The model under review builds one solid part; all positions refer to its coordinate system, in mm. Round coordinates to 2 decimals unless told otherwise and drop trailing zeros. Loops run counter-clockwise (first coordinate to the right, second up) from the corner with the lowest first, then second, coordinate; pieces in that order, holes last. Notation, with made-up numbers: M 47,-33 L 65,-33 A17 ccw 65,0 Z; hole C 18.25,48 d9. An arc over 180 degrees is marked long. Return JSON: item names as keys, results as strings. Group by question number.
Q1. To check wall thickness, follow line 1 along Y through (x, z) = (0, 7.5); line 2 along X through (y, z) = (3.5, 22.5); line 3 along X through (y, z) = (-24, 10.5). State the ranges of each line that lie inside material, in increasing order.
Q2. Consider section D-D (z = 8). State the section outline as (x, y) points.
Q3. Clearance check with flat-ended pins moving along their axes: pin 1 Ø6 at (y, z) = (-13, 22) entering from +X; pin 2 Ø4 at (x, y) = (10.5, 21) entering from -Z; pin 3 Ø5 at (x, y) = (0, 0) entering from -Z; pin 4 Ø1.5 at (y, z) = (-4, 24.5) entering from -X. State where each tip first meets the part, or that it passes through.
Q4. Consider section C-C (z = 15). State the section outline as (x, y) points.
Q5. Consider section A-A (x = 0). State the section outline as (y, z) points, and give its area (3 significant figures).
Q6. Draft analysis for pull direction Y (two halves, no side actions). For faces 1 (the face through (0, 6, 0)), 2 (the face through (0.28, -21.18, 7.04)), 3 (the face through (-0.878, -3.954, 14.79)), 4 (the face through (-21.18, -0.28, 7.04)), state which applies: pulls with the +Y half, pulls with the -Y half, needs draft (parallel to the pull), parting line crosses it, or undercut.
from build123d import *

# Parameters (mm, degrees)
F2_R     = 4.05
F3_DEPTH = 30
F4_R     = 17.5
F5_DEPTH = 25


with BuildPart() as f1:
    # F0 (on Front) → F1 (revolve)
    with BuildSketch(Plane.XZ):
        Polygon((-12.5, 30), (-35, 0), (0, 0), (0, 30), align=None)
    revolve(axis=Axis((0, 0, 15), (0, 0, 1)))

    # F2 (on Top) → F3 (cut)
    with BuildSketch(Plane.XY):
        Circle(F2_R)
    extrude(amount=F3_DEPTH, mode=Mode.SUBTRACT)

    # F4 (on Top) → F5 (cut)
    with BuildSketch(Plane.XY):
        with Locations((0, 38.677964)):
            Circle(F4_R)
        with Locations((-38.677964, 0)):
            Circle(F4_R)
        with Locations((0, -38.677964)):
            Circle(F4_R)
        with Locations((38.677964, 0)):
            Circle(F4_R)
    extrude(amount=F5_DEPTH, mode=Mode.SUBTRACT)


solid = f1.part
Values:
{
 "1": {"line 1": "y = -21.18 to -4.05, 4.05 to 21.18", "line 2": "x = -17.78 to -2.04, 2.04 to 17.78", "line 3": "x = -12.64 to -9.53, 9.53 to 12.64"},
 "2": {"outline": "M -26.25,-12.32 A29 ccw -12.32,-26.25 A17.5 cw 12.32,-26.25 A29 ccw 26.25,-12.32 A17.5 cw 26.25,12.32 A29 ccw 12.32,26.25 A17.5 cw -12.32,26.25 A29 ccw -26.25,12.32 A17.5 cw Z; hole C 0,0 d8.1"},
 "3": {"pin 1": "stops at x = 16.93", "pin 2": "stops at z = 0", "pin 3": "passes through", "pin 4": "stops at x = -16.74"},
 "4": {"outline": "M -22.67,-7.07 A23.75 ccw -7.07,-22.67 A17.5 cw 7.07,-22.67 A23.75 ccw 22.67,-7.07 A17.5 cw 22.67,7.07 A23.75 ccw 7.07,22.67 A17.5 cw -7.07,22.67 A23.75 ccw -22.67,7.07 A17.5 cw Z; hole C 0,0 d8.1"},
 "5": {"outline": "M -21.18,0 L -4.05,0 L -4.05,30 L -12.5,30 L -21.18,18.43 Z; M 4.05,0 L 21.18,0 L 21.18,18.43 L 12.5,30 L 4.05,30 Z", "area": "927 mm2"},
 "6": {"face 1": "needs draft", "face 2": "pulls with the -Y half", "face 3": "undercut", "face 4": "undercut"}
}
